For this review, take the finished solid that the model builds, in its own axes (mm). A direction names the side the tool comes from. Coordinates: 2 decimals unless noted, no trailing zeros. Write each loop counter-clockwise with the first axis right and the second up, starting at its lowest first coordinate (ties: lowest second). Pieces come first, ordered by that corner, then holes. Notation, with made-up numbers: (-21, 72.25) - (14, 72.25) arc R13 cw to (14, 80.25) - close; hole circle Ø6 at (21, -39.75). An arc over 180 degrees is marked (long way). Use one line per item in the form item = value. Start each with the question number.
1) Insertion check: P1, Ø7, axis at x = 0, z = 7.5, coming from the -Y side; P2, Ø4, axis at x = -15, y = 0, coming from the +Z side. Each pin has a flat end and moves straight along its axis. Give the tip position at first contact, or say it passes through.
2) We need section B-B (x = 0). Give the boundary of the cut face in (y, z), plus the area to 3 significant figures.
3) Tool access review of faces 1 (the flat face through (-4, 3, 7)), 2 (the flat face through (0, 10, 3)): name each direction out of +Z, -Z, +X, -X, +Y, -Y from which nothing blocks a thin tool from reaching the whole face with its end or side.
4) Mouldability with a two-part tool opening along X and no side actions: class faces 3 (the flat face through (0, 3, 3)), 4 (the flat face through (0, 0, 12)), 5 (the flat face through (20, 0, 6)) as pulls with the +X half, pulls with the -X half, needs draft (parallel to the pull), parting line crosses it, or undercut.
5) We need section C-C (y = 0). Count the separate pieces of the cut face and the enclosed holes in it, plus the area to 3 significant figures.
6) For L1, parallel to Y at x = -15, z = 3.5; L2, parallel to Z at x = 0, y = -6.75; L3, parallel to X at y = 0.25, z = 4.5, list the stretches that pass through material, from the lowest coordinate up. Write a range as from..to.
7) We need section A-A (z = 7.5). Give the boundary of the cut face in (x, y), plus the area to 3 significant figures.
8) We need section D-D (x = -15). Give the boundary of the cut face in (y, z).
```python
from build123d import *

# Parameters (mm, degrees)
F0_W     = 40
F0_H     = 20
F0_R     = 2.5
F0_W_2   = 8
F0_H_2   = 4
F1_DEPTH = 12
F2_DEPTH = 3
F3_R     = 2.75
F4_DEPTH = 25
F5_SIZE  = 2
F6_SIZE  = 1
F7_SIZE  = 0.49999


# Not quite as in the source:
# - a fillet or chamfer is up to 0.001 mm smaller than in the source, because OpenCascade refuses the exact size


with BuildPart() as f1:
    # F0 (on Top) → F1 (new body)
    with BuildSketch(Plane.XY):
        Rectangle(F0_W, F0_H)
        with Locations((-15, 0)):
            Circle(F0_R, mode=Mode.SUBTRACT)
        with Locations((0, 3)):
            Rectangle(F0_W_2, F0_H_2, mode=Mode.SUBTRACT)
        with Locations((15, 0)):
            Circle(F0_R, mode=Mode.SUBTRACT)
    extrude(amount=F1_DEPTH)

    # F0 (on Top) → F2 (join)
    with BuildSketch(Plane.XY):
        with Locations((0, 3)):
            Rectangle(F0_W_2, F0_H_2)
    extrude(amount=F2_DEPTH)

    # F3 (on face) → F4 (cut)
    with BuildSketch(Plane.XZ.offset(10)):
        with Locations((0, 7.5)):
            Circle(F3_R)
    extrude(amount=-F4_DEPTH, mode=Mode.SUBTRACT)

    # F5
    f5_edges = [f1.edges().sort_by_distance(p)[0] for p in [
        (-17.5, 0, 12),
        (12.5, 0, 12),
    ]]
    chamfer(f5_edges, length=F5_SIZE)

    # F6
    f6_edges = [f1.edges().sort_by_distance(p)[0] for p in [
        (-2.75, 10, 7.5),
        (-17.5, 0, 0),
        (12.5, 0, 0),
        (-2.75, -10, 7.5),
    ]]
    chamfer(f6_edges, length=F6_SIZE)

    # F7 (size 0.5 in the source; OpenCascade refuses exactly that, so slightly less here)
    f7_edges = [f1.edges().sort_by_distance(p)[0] for p in [
        (0, 10, 12),
        (20, 0, 12),
        (0, -10, 12),
        (-20, 0, 12),
        (-20, 10, 6),
        (20, 10, 6),
        (20, -10, 6),
        (-20, -10, 6),
    ]]
    chamfer(f7_edges, length=F7_SIZE)


solid = f1.part
```
Determined:
q1.P1 = -9.75
q1.P2 = through
q2.outline = (-10, 0) - (10, 0) - (10, 3.75) - (9, 4.75) - (5, 4.75) - (5, 3) - (1, 3) - (1, 4.75) - (-9, 4.75) - (-10, 3.75) - close; (-10, 11.25) - (-9, 10.25) - (1, 10.25) - (1, 12) - (-9.5, 12) - (-10, 11.5) - close; (5, 10.25) - (9, 10.25) - (10, 11.25) - (10, 11.5) - (9.5, 12) - (5, 12) - close
q2.area = 114 mm²
q3.face_1 = +Z
q3.face_2 = +Z, -Z, +X, -X, +Y
q4.face_3 = undercut
q4.face_4 = needs draft
q4.face_5 = pulls with the +X half
q5.separate_pieces = 3
q5.enclosed_holes = 1
q5.area = 326 mm²
q6.L1 = -10..-2.5, 2.5..10
q6.L2 = 0..4.75, 10.25..12
q6.L3 = -20..-17.49, -12.51..12.51, 17.49..20
q7.outline = (-20, -9.5) - (-19.5, -10) - (-3.75, -10) - (-2.75, -9) - (-2.75, 1) - (-4, 1) - (-4, 5) - (-2.75, 5) - (-2.75, 9) - (-3.75, 10) - (-19.5, 10) - (-20, 9.5) - close; (2.75, -9) - (3.75, -10) - (19.5, -10) - (20, -9.5) - (20, 9.5) - (19.5, 10) - (3.75, 10) - (2.75, 9) - (2.75, 5) - (4, 5) - (4, 1) - (2.75, 1) - close; hole circle Ø5 at (-15, 0); hole circle Ø5 at (15, 0)
q7.area = 638 mm²
q8.outline = (-10, 0) - (-3.5, 0) - (-2.5, 1) - (-2.5, 10) - (-4.5, 12) - (-9.5, 12) - (-10, 11.5) - close; (2.5, 1) - (3.5, 0) - (10, 0) - (10, 11.5) - (9.5, 12) - (4.5, 12) - (2.5, 10) - close
